Source: CAD feature listing. Evaluate the final solid. Frame: model axes, mm. A direction names the side the tool comes from. Coordinates: 2 decimals unless noted, no trailing zeros. Order: outer loops, then holes, each group sorted by start corner. A loop starts at its lowest first (then second) coordinate and runs counter-clockwise, first axis right, second up.
```python
from build123d import *

# Parameters (mm, degrees)
F0_W     = 130
F0_H     = 90
F1_DEPTH = 70
F2_T     = -1
F3_R     = 0.49999


# Not quite as in the source:
# - a fillet or chamfer is up to 0.001 mm smaller than in the source, because OpenCascade refuses the exact size


with BuildPart() as f1:
    # F0 (on Top) → F1 (new body)
    with BuildSketch(Plane.XY):
        Rectangle(F0_W, F0_H)
    extrude(amount=F1_DEPTH)

    # F2
    f2_openings = [f1.faces().sort_by_distance(p)[0] for p in [
        (0, 0, 70),
    ]]
    offset(amount=F2_T, openings=f2_openings)

    # F3 (radius 0.5 in the source; OpenCascade refuses exactly that, so slightly less here)
    f3_edges = [f1.edges().sort_by_distance(p)[0] for p in [
        (-65, -45, 35),
        (65, -45, 35),
        (0, -45, 0),
        (0, -45, 70),
        (-65, 45, 35),
        (-65, 0, 0),
        (-65, 0, 70),
        (65, 45, 35),
        (64, 44, 35.5),
        (-64, 44, 35.5),
        (-64, 0, 70),
        (-64, 0, 1),
        (0, 45, 70),
        (65, 0, 0),
        (65, 0, 70),
        (0, 45, 0),
        (64, -44, 35.5),
        (-64, -44, 35.5),
        (0, -44, 1),
        (0, -44, 70),
        (0, 44, 1),
        (0, 44, 70),
        (64, 0, 1),
        (64, 0, 70),
    ]]
    fillet(f3_edges, radius=F3_R)


solid = f1.part
```
Q1. Material intervals for line 1 along X through (y, z) = (-4.5, 54); line 2 along Y through (x, z) = (55, 7); line 3 along Z through (x, y) = (22.5, 25), sorted ascending.
Solutions:
line 1: x = -65 to -64, 64 to 65
line 2: y = -45 to -44, 44 to 45
line 3: z = 0 to 1
Q2. Pin query (flat end, axial travel): P1, Ø1, axis at x = -36.5, y = 8.5, coming from the +Z side. Return the tip coordinate at first contact, or that it passes through.
Solutions:
P1: stops at z = 1
Q3. Set-up query: faces 1 (the flat face through (-1, 45, 35)), 2 (the flat face through (-1, -44, 35)). Return all of +Z, -Z, +X, -X, +Y, -Y with unobstructed straight access to the full face (end or side cutting, diameter ignored); none if empty.
Solutions:
face 1: +Z, -Z, +X, -X, +Y
face 2: +Z
Q4. Section query B-B on z = 38.5. Output: boundary loops of the cut face in (x, y), plus the area to 3 significant figures.
Solutions:
outline: (-65, -44.5) arc R0.5 ccw to (-64.5, -45) - (64.5, -45) arc R0.5 ccw to (65, -44.5) - (65, 44.5) arc R0.5 ccw to (64.5, 45) - (-64.5, 45) arc R0.5 ccw to (-65, 44.5) - close; hole (-64, -43.5) arc R0.5 ccw to (-63.5, -44) - (63.5, -44) arc R0.5 ccw to (64, -43.5) - (64, 43.5) arc R0.5 ccw to (63.5, 44) - (-63.5, 44) arc R0.5 ccw to (-64, 43.5) - close
area: 436 mm2
Q5. Pull-direction query (Y, two-part tool) for faces 3 (the flat face through (-1, -45, 35)), 4 (the flat face through (-1, 44, 35)), 5 (the flat face through (65, -1, 35)); classes: pulls with the +Y half, pulls with the -Y half, needs draft (parallel to the pull), parting line crosses it, or undercut.
Solutions:
face 3: pulls with the -Y half
face 4: undercut
face 5: needs draft
